Autodesk Inventor part; units mm, degrees
ref_plane "YZ Plane" through (0, 0, 0) normal (1, 0, 0) x (0, 1, 0)
ref_plane "XZ Plane" through (0, 0, 0) normal (0, 1, 0) x (-1, 0, 0)
ref_plane "XY Plane" through (0, 0, 0) normal (0, 0, 1) x (1, 0, 0)
sketch "Sketch2" plane through (0, 0, 0) normal (0, 1, 0) x (-1, 0, 0)
  line L0 (-48.26, 44.5) -> (48.26, 44.5)
  line L1 (48.26, 44.5) -> (48.26, -44.5)
  line L2 (48.26, -44.5) -> (-48.26, -44.5)
  line L3 (-48.26, -44.5) -> (-48.26, 44.5)
  line L4 (-48.26, 44.5) -> (48.26, -44.5) construction
  line L5 (48.26, 44.5) -> (-48.26, -44.5) construction
  point P0 (0, 0)
  dimension "d0" = 96.52
  dimension "d1" = 89
extrude "Extrusion1" add sketch "Sketch2" along normal blind 5
sketch "Sketch3" plane through (0, 5, 0) normal (0, 1, 0) x (1, 0, 0)
  line L0 (48.26, 44.5) -> (-48.26, 44.5) construction
  line L1 (-15, 44.5) -> (-5, 44.5)
  line L2 (-5, 44.5) -> (-5, 41.5)
  line L3 (-5, 41.5) -> (-15, 41.5)
  line L4 (-15, 41.5) -> (-15, 44.5)
  line L5 (0, 62.3) -> (0, -62.3) construction
  point P0 (0, 0)
  dimension "d4" = 10
  dimension "d5" = 3
  dimension "d6" = 5
extrude "Extrusion2" cut sketch "Sketch3" against normal through all
pattern_linear "Rectangular Pattern1" count 2 spacing 20 along (-1, 0, 0) count 2 spacing 40 along (1, 0, 0) of "Extrusion2"
mirror "Mirror1" about plane through (0, 0, 0) normal (0, 0, 1) of "Extrusion2", "Rectangular Pattern1"
sketch "Sketch4" plane through (0, 5, 0) normal (0, 1, 0) x (1, 0, 0)
  line L0 (-48.26, 44.5) -> (-48.26, -44.5) construction
  line L1 (-48.26, 5) -> (-45.26, 5)
  line L2 (-45.26, 5) -> (-45.26, 15)
  line L3 (-45.26, 15) -> (-48.26, 15)
  line L4 (-48.26, 15) -> (-48.26, 5)
  line L5 (67.564, 0) -> (-67.564, 0) construction
  point P0 (0, 0)
  dimension "d15" = 3
  dimension "d16" = 10
  dimension "d17" = 5
extrude "Extrusion3" cut sketch "Sketch4" against normal through all
pattern_linear "Rectangular Pattern2" count 2 spacing 20 along (0, 0, -1) count 2 spacing 40 along (0, 0, 1) of "Extrusion3"
mirror "Mirror2" about plane through (0, 0, 0) normal (1, 0, 0) of "Extrusion3", "Rectangular Pattern2"
sketch "Sketch5" plane through (0, 5, 0) normal (0, 1, 0) x (1, 0, 0)
  line L0 (-36.26, 32.5) -> (-30.26, 32.5)
  line L1 (-30.26, 32.5) -> (-30.26, 28.5)
  line L2 (-30.26, 28.5) -> (-36.26, 28.5)
  line L3 (-36.26, 28.5) -> (-36.26, 32.5)
  line L4 (-35, 44.5) -> (-48.26, 44.5) construction
  line L5 (-48.26, 25) -> (-48.26, 15) construction
  point P0 (0, 0)
  dimension "d26" = 6
  dimension "d27" = 4
  dimension "d28" = 12
  dimension "d29" = 12
extrude "Extrusion4" cut sketch "Sketch5" against normal through all
equation "\"d0\" = Module_Width"
equation "\"d1\" = Module_Height"
equation "\"d2\" = Module_Back_Thickness"
equation "\"d4\" = Module_Case_SlotWidth"
equation "\"d5\" = Module_Case_SlotDepth"
equation "\"d6\" = 0.5 * Module_Case_SlotWidth"
equation "\"d7\" = ModuleBottomThickness"
equation "\"d11\" = 2 * Module_Case_SlotWidth"
equation "\"d14\" = 4 * Module_Case_SlotWidth"
equation "\"d15\" = Module_Case_SlotDepth"
equation "\"d16\" = Module_Case_SlotWidth"
equation "\"d17\" = 0.5 * Module_Case_SlotWidth"
equation "\"d18\" = ModuleBottomThickness"
equation "\"d22\" = 2 * Module_Case_SlotWidth"
equation "\"d25\" = 4 * Module_Case_SlotWidth"
equation "\"d26\" = Module_Connector_Width"
equation "\"d27\" = Module_Connector_Depth"
equation "\"d30\" = ModuleBottomThickness"
equation "\"ModuleBottomThickness\" = 5"
equation "\"RackWidth\" = 482.6"
equation "\"U\" = 44.5"
equation "\"Module_Width\" = 96.52"
equation "\"Module_Height\" = 89"
equation "\"Module_Case_Thickness\" = 3"
equation "\"Module_Back_Thickness\" = 5"
equation "\"Module_Case_SlotDepth\" = 3"
equation "\"Module_Case_SlotWidth\" = 10"
equation "\"Module_Connector_Width\" = 6"
equation "\"Module_Connector_Depth\" = 4"
equation "\"Module_StatusIndicatorDiameter\" = 5"
equation "\"Module_Case_BottomSlotDepth\" = 5"
properties part number "BackPlateBase" material "Wood (Birch)"
Geometry check sheet. Reference: the model listing, model coordinates, mm. A direction names the side the tool comes from. Round coordinates to 2 decimals unless told otherwise and drop trailing zeros. Order: outer loops, then holes, each group sorted by start corner. A loop starts at its lowest first (then second) coordinate and runs counter-clockwise, first axis right, second up. Notation, with made-up numbers: (0, -7) -> (22, -7) arc R21 ccw to (22, 31) -> close; hole circle Ø7 at (14.5, 18.25). An arc over 180 degrees is marked (long way). Return JSON: item names as keys, results as strings. Group by question number.
Q1. Section check B-B, the plane z = 32.5. Record the boundary of the cut face in (x, y).
Q2. Tool access check on faces 1 (the flat face through (-33, 3, -28.5)), 2 (the flat face through (15, 3, 43)), 3 (the flat face through (-5, 3, -43)), 4 (the flat face through (45.26, 3, 30)), 5 (the flat face through (-47, 3, -35)). Record the directions out of +Z, -Z, +X, -X, +Y, -Y that give a thin tool (end or side, any length) a straight path to the whole face; none if there is none.
Q3. Material ranges on probe 1 along Z at (x, y) = (-33, 2.1); probe 2 along X at (y, z) = (3.85, -29); probe 3 along Z at (x, y) = (-30, 0.7), recorded low to high. Write a range as from..to.
Q4. Section check A-A, the plane x = -26.5. Record the boundary of the cut face in (y, z).
Q5. Gauge pin test, flat ends, axial feed: pin 1 (1.5 mm diameter, centred on y = 0.5, z = 11, fed in from +X); pin 2 (1.5 mm diameter, centred on x = 28.5, z = 28, fed in from -Y); pin 3 (1.5 mm diameter, centred on x = -34, y = 1.5, fed in from +Z). Record the tip position at first contact, or that the pin passes through.
Q6. Release check for a two-part mould opening along Z. For faces 6 (the flat face through (45.26, 3, 10)), 7 (the flat face through (5, 3, -43)), 8 (the flat face through (47, 3, 5)), 9 (the flat face through (-30, 3, -41.5)) record: released by +Z, released by -Z, zero draft, split by the parting line, or undercut.
Numbers:
{
 "1": {"outline": "(-45.26, 0) -> (45.26, 0) -> (45.26, 5) -> (-45.26, 5) -> close"},
 "2": {"face 1": "+Y, -Y", "face 2": "+Z, +Y, -Y", "face 3": "-Z, +Y, -Y", "face 4": "+X, +Y, -Y", "face 5": "-X, +Y, -Y"},
 "3": {"probe 1": "-41.5..-32.5, -28.5..41.5", "probe 2": "-45.26..-36.26, -30.26..45.26", "probe 3": "-41.5..41.5"},
 "4": {"outline": "(0, -41.5) -> (5, -41.5) -> (5, 41.5) -> (0, 41.5) -> close"},
 "5": {"pin 1": "x = 45.26", "pin 2": "y = 0", "pin 3": "z = 41.5"},
 "6": {"face 6": "undercut", "face 7": "zero draft", "face 8": "undercut", "face 9": "released by -Z"}
}
